from build123d import *

# Parameters (mm, degrees)
ESQUISSE2_R                  = 13
BOSS_EXTRU_1_DEPTH           = 25
ESQUISSE3_R                  = 9
ENL_V_MAT_EXTRU_1_DEPTH      = 32.032241298
ESQUISSE4_R                  = 11
ENL_V_MAT_EXTRU_2_DEPTH      = 7
ESQUISSE6_R                  = 0.75
BOSS_EXTRU_2_DEPTH           = 25
R_P_TITION_CIRCULAIRE1_COUNT = 8
SYM_TRIE2_COPY_1_SKETCH_R    = 0.75
SYM_TRIE2_COPY_1_DEPTH       = 25
SYM_TRIE2_COPY_2_SKETCH_R    = 0.75
SYM_TRIE2_COPY_2_DEPTH       = 25
SYM_TRIE2_COPY_3_SKETCH_R    = 0.75
SYM_TRIE2_COPY_3_DEPTH       = 25
SYM_TRIE2_COPY_4_SKETCH_R    = 0.75
SYM_TRIE2_COPY_4_DEPTH       = 25
SYM_TRIE2_COPY_5_SKETCH_R    = 0.75
SYM_TRIE2_COPY_5_DEPTH       = 25
SYM_TRIE2_COPY_6_SKETCH_R    = 0.75
SYM_TRIE2_COPY_6_DEPTH       = 25
SYM_TRIE2_COPY_7_SKETCH_R    = 0.75
SYM_TRIE2_COPY_7_DEPTH       = 25


with BuildPart() as part:
    # Esquisse2 → Boss.-Extru.1 (new body)
    with BuildSketch(Plane(origin=(0, 0, 0), x_dir=(1, 0, 0), z_dir=(0, 1, 0))):
        with Locations(Location((0, 0, 0), (0, 0, 270))):
            Circle(ESQUISSE2_R)
    boss_extru_1 = extrude(amount=BOSS_EXTRU_1_DEPTH)

    # Esquisse3 → Enlèv. mat.-Extru.1 (cut, through all)
    with BuildSketch(Plane.XZ):
        with Locations(Location((0, 0, 0), (0, 0, 270))):
            Circle(ESQUISSE3_R)
    enl_v_mat_extru_1 = extrude(amount=-ENL_V_MAT_EXTRU_1_DEPTH, mode=Mode.SUBTRACT)

    # Esquisse4 → Enlèv. mat.-Extru.2 (cut)
    with BuildSketch(Plane.XZ):
        with Locations(Location((0, 0, 0), (0, 0, 270))):
            Circle(ESQUISSE4_R)
    enl_v_mat_extru_2 = extrude(amount=-ENL_V_MAT_EXTRU_2_DEPTH, mode=Mode.SUBTRACT)

    # Esquisse6 → Boss.-Extru.2 (add)
    with BuildSketch(Plane(origin=(0, 0, 0), x_dir=(-1, 0, 0), z_dir=(0, -1, 0))):
        with Locations((-13, 0)):
            Circle(ESQUISSE6_R)
    boss_extru_2 = extrude(amount=-BOSS_EXTRU_2_DEPTH)

    # Répétition circulaire1: Boss.-Extru.2 ×8 about axis
    r_p_tition_circulaire1_axis = Axis((0, 0, 0), (0, 1, 0))
    for i in range(1, R_P_TITION_CIRCULAIRE1_COUNT):
        add(boss_extru_2.rotate(r_p_tition_circulaire1_axis, i * 360 / R_P_TITION_CIRCULAIRE1_COUNT))

    # Symétrie2: Boss.-Extru.1, Enlèv. mat.-Extru.1, Enlèv. mat.-Extru.2, Boss.-Extru.2 across plane
    add(boss_extru_1.mirror(Plane.ZX.offset(25)))
    add(enl_v_mat_extru_1.mirror(Plane.ZX.offset(25)), mode=Mode.SUBTRACT)
    add(enl_v_mat_extru_2.mirror(Plane.ZX.offset(25)), mode=Mode.SUBTRACT)
    add(boss_extru_2.mirror(Plane.ZX.offset(25)))

    # Symétrie2 copy 1 sketch → Symétrie2 copy 1 (add)
    with BuildSketch(Plane(origin=(0, 50, 0), x_dir=(-0.7071067811865476, 0, 0.7071067811865475), z_dir=(0, 1, 0))):
        with Locations((-13, 0)):
            Circle(SYM_TRIE2_COPY_1_SKETCH_R)
    extrude(amount=-SYM_TRIE2_COPY_1_DEPTH)

    # Symétrie2 copy 2 sketch → Symétrie2 copy 2 (add)
    with BuildSketch(Plane.ZX.offset(50)):
        with Locations((-13, 0)):
            Circle(SYM_TRIE2_COPY_2_SKETCH_R)
    extrude(amount=-SYM_TRIE2_COPY_2_DEPTH)

    # Symétrie2 copy 3 sketch → Symétrie2 copy 3 (add)
    with BuildSketch(Plane(origin=(0, 50, 0), x_dir=(0.7071067811865475, 0, 0.7071067811865476), z_dir=(0, 1, 0))):
        with Locations((-13, 0)):
            Circle(SYM_TRIE2_COPY_3_SKETCH_R)
    extrude(amount=-SYM_TRIE2_COPY_3_DEPTH)

    # Symétrie2 copy 4 sketch → Symétrie2 copy 4 (add)
    with BuildSketch(Plane(origin=(0, 50, 0), x_dir=(1, 0, 0), z_dir=(0, 1, 0))):
        with Locations((-13, 0)):
            Circle(SYM_TRIE2_COPY_4_SKETCH_R)
    extrude(amount=-SYM_TRIE2_COPY_4_DEPTH)

    # Symétrie2 copy 5 sketch → Symétrie2 copy 5 (add)
    with BuildSketch(Plane(origin=(0, 50, 0), x_dir=(0.7071067811865477, 0, -0.7071067811865475), z_dir=(0, 1, 0))):
        with Locations((-13, 0)):
            Circle(SYM_TRIE2_COPY_5_SKETCH_R)
    extrude(amount=-SYM_TRIE2_COPY_5_DEPTH)

    # Symétrie2 copy 6 sketch → Symétrie2 copy 6 (add)
    with BuildSketch(Plane(origin=(0, 50, 0), x_dir=(0, 0, -1), z_dir=(0, 1, 0))):
        with Locations((-13, 0)):
            Circle(SYM_TRIE2_COPY_6_SKETCH_R)
    extrude(amount=-SYM_TRIE2_COPY_6_DEPTH)

    # Symétrie2 copy 7 sketch → Symétrie2 copy 7 (add)
    with BuildSketch(Plane(origin=(0, 50, 0), x_dir=(-0.7071067811865474, 0, -0.7071067811865477), z_dir=(0, 1, 0))):
        with Locations((-13, 0)):
            Circle(SYM_TRIE2_COPY_7_SKETCH_R)
    extrude(amount=-SYM_TRIE2_COPY_7_DEPTH)


solid = part.part
Part model, mm, in its own coordinate system. A direction names the side the tool comes from. Give positions to 0.01 mm unless a question says otherwise; leave off trailing zeros. Write each loop counter-clockwise with the first axis right and the second up, starting at its lowest first coordinate (ties: lowest second). Pieces come first, ordered by that corner, then holes.
1) Pin check, flat tips, straight feed: pin 1 (3 mm diameter, centred on x = 6, y = 30, fed in from -Z); pin 2 (5 mm diameter, centred on x = -8, z = -2, fed in from +Y); pin 3 (2 mm diameter, centred on x = 3.5, y = 14.5, fed in from +Z); pin 4 (6.5 mm diameter, centred on x = 2, z = -3.5, fed in from -Y). Stop position of each tip, or through.
Resolved:
pin 1: stops at z = -12.2
pin 2: stops at y = 43
pin 3: stops at z = 12.76
pin 4: passes through
2) Cut at A-A on z = 0. Write the cut outline in (x, y), then the cut area to 3 significant figures.
Resolved:
outline: (-13.75, 0) - (-11, 0) - (-11, 7) - (-9, 7) - (-9, 43) - (-11, 43) - (-11, 50) - (-13.75, 50) - close; (9, 7) - (11, 7) - (11, 0) - (13.75, 0) - (13.75, 50) - (11, 50) - (11, 43) - (9, 43) - close
area: 419 mm2
3) Cut at C-C on x = 7.75. Write the cut outline in (y, z), then the cut area to 3 significant figures.
Resolved:
outline: (0, -10.44) - (50, -10.44) - (50, -7.81) - (43, -7.81) - (43, -4.58) - (7, -4.58) - (7, -7.81) - (0, -7.81) - close; (0, 7.81) - (7, 7.81) - (7, 4.58) - (43, 4.58) - (43, 7.81) - (50, 7.81) - (50, 10.44) - (0, 10.44) - close
area: 496 mm2
4) Probe L1, parallel to Z at x = 0, y = 15.5; L2, parallel to X at y = 5.25, z = 0. List the from-to ranges inside material, lowest first.
Resolved:
L1: z = -13.75 to -9, 9 to 13.75
L2: x = -13.75 to -11, 11 to 13.75
5) Cut at B-B on y = 26. Write the cut outline in (x, z), then the cut area to 3 significant figures.
Resolved:
outline: (-12.98, -0.75) arc R13 ccw to (-9.71, -8.65) arc R0.75 ccw (long way) to (-8.65, -9.71) arc R13 ccw to (-0.75, -12.98) arc R0.75 ccw (long way) to (0.75, -12.98) arc R13 ccw to (8.65, -9.71) arc R0.75 ccw (long way) to (9.71, -8.65) arc R13 ccw to (12.98, -0.75) arc R0.75 ccw (long way) to (12.98, 0.75) arc R13 ccw to (9.71, 8.65) arc R0.75 ccw (long way) to (8.65, 9.71) arc R13 ccw to (0.75, 12.98) arc R0.75 ccw (long way) to (-0.75, 12.98) arc R13 ccw to (-8.65, 9.71) arc R0.75 ccw (long way) to (-9.71, 8.65) arc R13 ccw to (-12.98, 0.75) arc R0.75 ccw (long way) to start; hole circle Ø18 at (0, 0)
area: 284 mm2
6) Which spindle directions (+Z, -Z, +X, -X, +Y, -Y) get a long thin tool onto all of the face, cutting with end or side? Do faces 5 (the face through (9.711, 25.35, 9.734)), 6 (the face through (-9, 7, -2)), 7 (the face through (-10.74, 46.55, 2.38)). Say none if no direction does.
Resolved:
face 5: +Y, -Y
face 6: -Y
face 7: +Y
7) Two-plate mould, pull along X, no slides. Class faces 1 (the face through (-0.02, 25.35, 13.75)), 2 (the face through (-9.711, 25.35, -9.734)), 3 (the face through (-12, 25, 5)), 4 (the face through (11.3, 0, -1.1)): released by +X, released by -X, zero draft, split by the parting line, or undercut.
Resolved:
face 1: split by the parting line
face 2: undercut
face 3: released by -X
face 4: zero draft
